```python
from build123d import *

# Parameters (mm, degrees)
BOSS_EXTRUDE1_DEPTH = 12.7
SKETCH2_R           = 7.9502
CUT_EXTRUDE1_DEPTH  = 42.311923389
SKETCH3_R           = 3.175
CUT_EXTRUDE2_DEPTH  = 42.311923389


with BuildPart() as part:
    # Sketch1 → Boss-Extrude1 (new body)
    with BuildSketch(Plane(origin=(0, 0, 0), x_dir=(1, 0, 0), z_dir=(0, 1, 0))):
        with BuildLine():
            Line((-25.4, 0), (25.4, 0))
            Line((25.4, 0), (25.4, 6.35))
            Line((25.4, 6.35), (13.49375, 6.35))
            Line((13.49375, 6.35), (13.49375, 16.51))
            ThreePointArc((13.49375, 16.51), (0, 30.00375), (-13.49375, 16.51))
            Line((-13.49375, 16.51), (-13.49375, 6.35))
            Line((-13.49375, 6.35), (-25.4, 6.35))
            Line((-25.4, 6.35), (-25.4, 0))
        make_face()
    extrude(amount=BOSS_EXTRUDE1_DEPTH)

    # Sketch2 → Cut-Extrude1 (cut, through all)
    with BuildSketch(Plane(origin=(0, 12.7, 0), x_dir=(1, 0, 0), z_dir=(0, 1, 0))):
        with Locations(Location((0, 15.375414513, 0), (0, 0, 270))):
            Circle(SKETCH2_R)
    extrude(amount=-CUT_EXTRUDE1_DEPTH, mode=Mode.SUBTRACT)

    # Sketch3 → Cut-Extrude2 (cut, through all)
    with BuildSketch(Plane.XY):
        with Locations((-19.05, 6.35)):
            Circle(SKETCH3_R)
        with Locations((19.05, 6.35)):
            Circle(SKETCH3_R)
    extrude(amount=-CUT_EXTRUDE2_DEPTH, mode=Mode.SUBTRACT)


solid = part.part
```
Source: CAD feature listing. Evaluate the final solid. Frame: model axes, mm. A direction names the side the tool comes from. Give positions to 0.01 mm unless a question says otherwise; leave off trailing zeros. Write each loop counter-clockwise with the first axis right and the second up, starting at its lowest first coordinate (ties: lowest second). Pieces come first, ordered by that corner, then holes.
1. Material intervals for line 1 along Y through (x, z) = (-19.05, -4.5) (3 decimals); line 2 along X through (y, z) = (8.75, -6); line 3 along Z through (x, y) = (1.5, 11), sorted ascending.
2. Access query for faces 1 (the face through (-3.04, 6.44, -8.03)), 2 (the face through (22, 8, -6.35)), 3 (the face through (-22, 4.8, -6.35)). Directions: +Z, -Z, +X, -X, +Y, -Y. A direction counts if a zero-diameter tool reaches every point of the face in a straight line with its end or side. Return the directions, or none.
3. First-contact query: pin 1 (1.5 mm diameter, centred on y = 4.5, z = -8.5, fed in from +X); pin 2 (7.5 mm diameter, centred on x = 19.05, y = 6.35, fed in from -Z); pin 3 (2 mm diameter, centred on y = 3, z = -26.5, fed in from +X); pin 4 (14.5 mm diameter, centred on x = 0, z = -15.38, fed in from -Y) (3 decimals). Flat tips, straight axial feed; report the tip coordinate or a pass-through.
4. Section query D-D (z = -20). Return the cut outline in (x, y).
5. Pull-direction query (Y, two-part tool) for faces 4 (the face through (0, 6, 0)), 5 (the face through (0, 12.7, -5)), 6 (the face through (-17.3, 9, -3.1)); classes: +Y half, -Y half, draft (parallel to the pull), parting line (faces both ways), or undercut.
6. Section query C-C (z = -2.5). Return the cut outline in (x, y) (3 decimals).
7. Section query A-A (y = 6.35). Count the separate pieces of the cut face and the enclosed holes in it, then the cut area to 3 significant figures.
8. Section query B-B (x = -19.05). Return the cut outline in (y, z) (3 decimals), then the cut area to 3 significant figures.
Output values:
1. line 1: y = 0 to 3.175, 9.525 to 12.7
1. line 2: x = -25.4 to -21.13, -16.97 to 16.97, 21.13 to 25.4
1. line 3: z = -29.92 to -23.18, -7.57 to 0
2. face 1: +Y, -Y
2. face 2: -Z, +X, +Y, -Y
2. face 3: -Z, -X, +Y, -Y
3. pin 1: stops at x = 13.49
3. pin 2: stops at z = -6.35
3. pin 3: stops at x = 10.06
3. pin 4: passes through
4. outline: (-13.03, 0) - (-6.47, 0) - (-6.47, 12.7) - (-13.03, 12.7) - close; (6.47, 0) - (13.03, 0) - (13.03, 12.7) - (6.47, 12.7) - close
5. face 4: draft
5. face 5: +Y half
5. face 6: undercut
6. outline: (-25.4, 0) - (25.4, 0) - (25.4, 12.7) - (-25.4, 12.7) - close; hole circle Ø6.35 at (-19.05, 6.35); hole circle Ø6.35 at (19.05, 6.35)
7. separate pieces: 3
7. enclosed holes: 1
7. area: 604 mm2
8. outline: (0, -6.35) - (3.175, -6.35) - (3.175, 0) - (0, 0) - close; (9.525, -6.35) - (12.7, -6.35) - (12.7, 0) - (9.525, 0) - close
8. area: 40.3 mm2
